```python
from build123d import *

# Parameters (mm, degrees)
MASS_DEPTH                = 6.35
SKETCH4_R                 = 9.271
CUT_EXTRUDE1_DEPTH        = 45.627810093
SKETCH3_W                 = 9.525
SKETCH3_H                 = 12.7
CUT_EXTRUDE2_DEPTH        = 45.627810093
F_6_32_TAPPED_HOLE1_D     = 2.7051
F_6_32_TAPPED_HOLE1_DEPTH = 152.4
F_6_32_TAPPED_HOLE1_TIP   = 0.81269403
CAVITY1_START             = -2.994165629
CAVITY1_OUTLINE_W         = 6.35
CAVITY1_OUTLINE_H         = 6.35
CAVITY1_DEPTH             = 6.35
CAVITY1_START_2           = 10.66280621
CAVITY1_2_OUTLINE_W       = 6.35
CAVITY1_2_OUTLINE_H       = 6.35
CAVITY1_2_DEPTH           = 6.35


# Read off the part's stored shape, not the designer's step: Cavity1
with BuildPart() as part:
    # Sketch1 → Mass (new body)
    with BuildSketch(Plane.XY):
        with BuildLine():
            Line((3.348333413, -17.092726624), (31.923333413, -17.092726624))
            Line((31.923333413, -17.092726624), (31.923333413, 30.532273376))
            Line((31.923333413, 30.532273376), (3.348333413, 30.532273376))
            Line((3.348333413, 30.532273376), (-11.189304159, 28.838055246))
            ThreePointArc((-11.189304159, 28.838055246), (-24.630570771, 17.379148263), (-19.157836039, 0.585596764))
            Line((-19.157836039, 0.585596764), (3.348333413, -17.092726624))
        make_face()
    extrude(amount=MASS_DEPTH)

    # Sketch4 → Cut-Extrude1 (cut, through all)
    with BuildSketch(Plane(origin=(0, 0, 0), x_dir=(-1, 0, 0), z_dir=(0, 0, -1))):
        with Locations((9.351666587, 13.069773376)):
            Circle(SKETCH4_R)
    extrude(amount=-CUT_EXTRUDE1_DEPTH, mode=Mode.SUBTRACT)

    # Sketch3 → Cut-Extrude2 (cut, through all)
    with BuildSketch(Plane(origin=(0, 0, 0), x_dir=(-1, 0, 0), z_dir=(0, 0, -1))):
        with Locations((-17.635833413, 30.532273376)):
            Rectangle(SKETCH3_W, SKETCH3_H)
        with Locations((-17.635833413, -17.092726624)):
            Rectangle(SKETCH3_W, SKETCH3_H)
    extrude(amount=-CUT_EXTRUDE2_DEPTH, mode=Mode.SUBTRACT)

    # #6-32 Tapped Hole1
    with Locations(Plane.XY.offset(6.35)):
        with Locations((10.764107125, -7.046000335), (4.47792784, 26.899367802), (-9.351666587, 13.069773376)):
            Hole(F_6_32_TAPPED_HOLE1_D / 2, depth=F_6_32_TAPPED_HOLE1_DEPTH)
            with Locations((0, 0, -(F_6_32_TAPPED_HOLE1_DEPTH + F_6_32_TAPPED_HOLE1_TIP / 2))):  # 118° drill point
                Cone(0, F_6_32_TAPPED_HOLE1_D / 2, F_6_32_TAPPED_HOLE1_TIP, mode=Mode.SUBTRACT)

    # Cavity1 outline → Cavity1 (cut)
    with BuildSketch(Plane(origin=(0, 0, 0), x_dir=(1, 0, 0), z_dir=(0, 1, 0)).offset(CAVITY1_START)):
        with Locations((6.523333416, -3.175)):
            Rectangle(CAVITY1_OUTLINE_W, CAVITY1_OUTLINE_H)
    extrude(amount=CAVITY1_DEPTH, mode=Mode.SUBTRACT)

    # Cavity1 2 outline → Cavity1 2 (cut)
    with BuildSketch(Plane(origin=(0, 0, 0), x_dir=(1, 0, 0), z_dir=(0, 1, 0)).offset(CAVITY1_START_2)):
        with Locations((6.523333416, -3.175)):
            Rectangle(CAVITY1_2_OUTLINE_W, CAVITY1_2_OUTLINE_H)
    extrude(amount=CAVITY1_2_DEPTH, mode=Mode.SUBTRACT)


solid = part.part
```
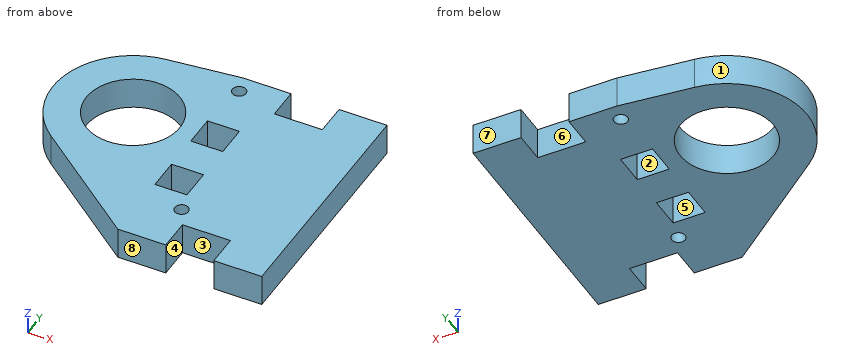
The model under review builds one solid part; all positions refer to its coordinate system, in mm. Face numbers are marked on the shaded views. A direction names the side the tool comes from. Round coordinates to 2 decimals unless told otherwise and drop trailing zeros. Write each loop counter-clockwise with the first axis right and the second up, starting at its lowest first coordinate (ties: lowest second). Pieces come first, ordered by that corner, then holes. Notation, with made-up numbers: (21, 47) - (37, 47) arc R27 cw to (37, 73) - close; hole circle Ø4 at (-9, 72). An arc over 180 degrees is marked (long way). Answer as CSV lines item,"result". Start each with the question number.
(1) To check wall thickness, follow line 1 (X direction, y = 12.5, z = 4.75); line 2 (Y direction, x = 3.5, z = 3) (3 decimals); line 3 (X direction, y = 18, z = 3). State the ranges of each line that lie inside material, in increasing order.
(2) Draft analysis for pull direction Y (two halves, no side actions). For the marked faces 1, 2 and 3, state which applies: pulls with the +Y half, pulls with the -Y half, needs draft (parallel to the pull), parting line crosses it, or undercut.
(3) We need section B-B on y = 9. State the section outline as (x, z) points.
(4) We need section A-A on y = 27.5. State the section outline as (x, z) points.
(5) For the marked faces 4, 5, 6, 7 and 8, list the 3-axis set-ups (+Z, -Z, +X, -X, +Y, -Y) from which the entire face can be reached by the end or side of a thin tool; tool diameter is ignored.
(6) For pin 1 Ø1 at (y, z) = (19.5, 1) entering from -X; pin 2 Ø3 at (y, z) = (0.5, 3) entering from -X, all flat-tipped, find the tip position at first contact; note any pin that passes through.
(7) We need section C-C on x = -9. State the section outline as (y, z) points, plus the area to 3 significant figures.
(8) We need section D-D on z = 2.5. State the section outline as (x, y) points (3 decimals).
Worked answers:
1,line 1,"-25.22 to -18.61, -0.1 to 3.35, 9.7 to 31.92"
1,line 2,"-17.093 to -2.994, 3.356 to 10.663, 17.013 to 25.965, 27.834 to 30.532"
1,line 3,"-24.44 to -17.2, -1.5 to 31.92"
2,face 1,"parting line crosses it"
2,face 2,"undercut"
2,face 3,"pulls with the -Y half"
3,outline,"(-24.7, 0) - (-17.68, 0) - (-17.68, 6.35) - (-24.7, 6.35) - close; (-1.02, 0) - (31.92, 0) - (31.92, 6.35) - (-1.02, 6.35) - close"
4,outline,"(-15.97, 0) - (3.27, 0) - (3.27, 6.35) - (-15.97, 6.35) - close; (5.69, 0) - (12.87, 0) - (12.87, 6.35) - (5.69, 6.35) - close; (22.4, 0) - (31.92, 0) - (31.92, 6.35) - (22.4, 6.35) - close"
5,face 4,"+Z, -Z, -Y"
5,face 5,"+Z, -Z"
5,face 6,"+Z, -Z, +Y"
5,face 7,"+Z, -Z, +X, -X, +Y"
5,face 8,"+Z, -Z, +X, -X, -Y"
6,pin 1,"x = -24.08"
6,pin 2,"x = -20.73"
7,outline,"(-7.39, 0) - (3.81, 0) - (3.81, 6.35) - (-7.39, 6.35) - close; (22.33, 0) - (29.09, 0) - (29.09, 6.35) - (22.33, 6.35) - close"
7,area,"114 mm²"
8,outline,"(-19.158, 0.586) - (3.348, -17.093) - (12.873, -17.093) - (12.873, -10.743) - (22.398, -10.743) - (22.398, -17.093) - (31.923, -17.093) - (31.923, 30.532) - (22.398, 30.532) - (22.398, 24.182) - (12.873, 24.182) - (12.873, 30.532) - (3.348, 30.532) - (-11.189, 28.838) arc R15.875 ccw to start; hole circle Ø18.542 at (-9.352, 13.07); hole circle Ø2.705 at (4.478, 26.899); hole (3.348, -2.994) - (9.698, -2.994) - (9.698, 3.356) - (3.348, 3.356) - close; hole (3.348, 10.663) - (9.698, 10.663) - (9.698, 17.013) - (3.348, 17.013) - close; hole circle Ø2.705 at (10.764, -7.046)"
